Verification items for the finished model (mm, model axes). Coordinates: 2 decimals unless noted, no trailing zeros. Order: outer loops, then holes, each group sorted by start corner. A loop starts at its lowest first (then second) coordinate and runs counter-clockwise, first axis right, second up. Notation, with made-up numbers: M 73.25,30.5 L 83.25,30.5 A17 ccw 83.25,58.5 Z; hole C -21.75,64.5 d9. An arc over 180 degrees is marked long. Return JSON: item names as keys, results as strings.
```python
from build123d import *

# Parameters (mm, degrees)
F0_R     = 4
F0_R_2   = 6
F1_DEPTH = 1.5


with BuildPart() as f1:
    # F0 (on Front) → F1 (new body, symmetric)
    with BuildSketch(Plane.XZ):
        with BuildLine():
            ThreePointArc((10, 210), (0, 220), (-10, 210))
            Line((-10, 210), (-10, -210))
            ThreePointArc((-10, -210), (0, -220), (10, -210))
            Line((10, -210), (10, 210))
        make_face()
        with Locations((0, -200)):
            Circle(F0_R, mode=Mode.SUBTRACT)
        Circle(F0_R_2, mode=Mode.SUBTRACT)
        with Locations((0, 200)):
            Circle(F0_R, mode=Mode.SUBTRACT)
    extrude(amount=F1_DEPTH, both=True)


solid = f1.part
```
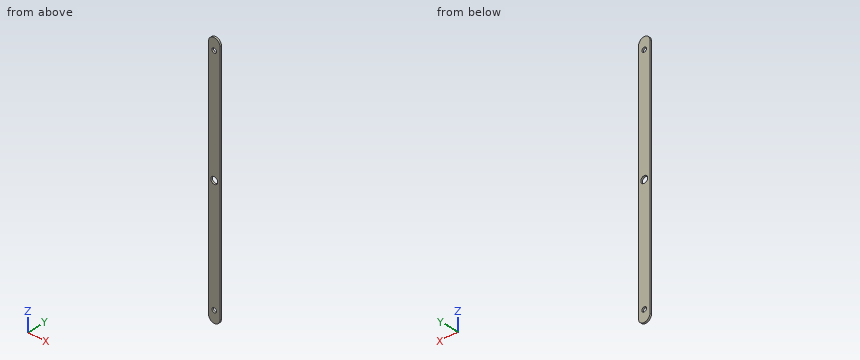
Q1. Material ranges on line 1 along Z through (x, y) = (0, 0.4); line 2 along Z through (x, y) = (2.5, 1.35); line 3 along Z through (x, y) = (7.5, 0.65), recorded low to high.
Values:
{"line 1": "-220 to -204, -196 to -6, 6 to 196, 204 to 220", "line 2": "-219.68 to -203.12, -196.88 to -5.45, 5.45 to 196.88, 203.12 to 219.68", "line 3": "-216.61 to 216.61"}
Q2. Cross-section at D-D, the plane z = -200. Record the boundary of the cut face in (x, y).
Values:
{"outline": "M -10,-1.5 L -4,-1.5 L -4,1.5 L -10,1.5 Z; M 4,-1.5 L 10,-1.5 L 10,1.5 L 4,1.5 Z"}
Q3. Go/stop test with flat-tipped pins: pin 1 (1.5 mm diameter, centred on x = -7, y = 0.5, fed in from +Z); pin 2 (7 mm diameter, centred on x = 0, z = 0, fed in from -Y); pin 3 (10.5 mm diameter, centred on x = 0, z = -200, fed in from +Y). Record where each tip stops, or that it passes through.
Values:
{"pin 1": "z = 217.81", "pin 2": "through", "pin 3": "y = 1.5"}
Q4. Cross-section at B-B, the plane x = 0. Record the boundary of the cut face in (y, z).
Values:
{"outline": "M -1.5,-220 L 1.5,-220 L 1.5,-204 L -1.5,-204 Z; M -1.5,-196 L 1.5,-196 L 1.5,-6 L -1.5,-6 Z; M -1.5,6 L 1.5,6 L 1.5,196 L -1.5,196 Z; M -1.5,204 L 1.5,204 L 1.5,220 L -1.5,220 Z"}
Q5. Cross-section at A-A, the plane z = 0. Record the boundary of the cut face in (x, y).
Values:
{"outline": "M -10,-1.5 L -6,-1.5 L -6,1.5 L -10,1.5 Z; M 6,-1.5 L 10,-1.5 L 10,1.5 L 6,1.5 Z"}
Q6. Cross-section at C-C, the plane y = 0.85. Record the boundary of the cut face in (x, z), and give its area (3 significant figures).
Values:
{"outline": "M -10,-210 A10 ccw 10,-210 L 10,210 A10 ccw -10,210 Z; hole C 0,0 d12; hole C 0,-200 d8; hole C 0,200 d8", "area": "8,500 mm^2"}
